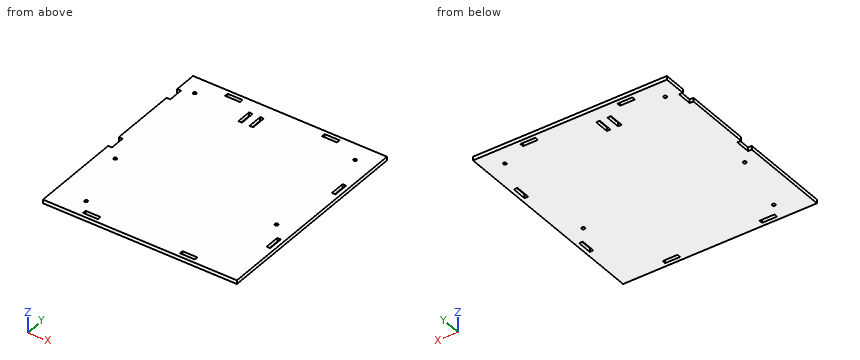
```python
from build123d import *

# Parameters (mm, degrees)
SKETCH1_W           = 260
SKETCH1_H           = 283
SKETCH1_W_2         = 20
SKETCH1_H_2         = 4.8
SKETCH1_W_3         = 4.8
SKETCH1_H_3         = 20
BOSS_EXTRUDE1_DEPTH = 5
SKETCH2_W           = 4.8
SKETCH2_H           = 20
CUT_EXTRUDE1_DEPTH  = 5
SKETCH3_R           = 2.1
CUT_EXTRUDE2_DEPTH  = 5
SKETCH4_R           = 2.1
CUT_EXTRUDE3_DEPTH  = 5
SKETCH5_R           = 2.1
CUT_EXTRUDE4_DEPTH  = 5
SKETCH6_R           = 2.1
CUT_EXTRUDE5_DEPTH  = 5
SKETCH7_W           = 5
SKETCH7_H           = 20
CUT_EXTRUDE6_DEPTH  = 10


with BuildPart() as part:
    # Sketch1 → Boss-Extrude1 (new body)
    with BuildSketch(Plane.XY):
        with Locations((-120, 136.5)):
            Rectangle(SKETCH1_W, SKETCH1_H)
        with Locations((-190, 2.5)):
            Rectangle(SKETCH1_W_2, SKETCH1_H_2, mode=Mode.SUBTRACT)
        with Locations((-60, 2.5)):
            Rectangle(SKETCH1_W_2, SKETCH1_H_2, mode=Mode.SUBTRACT)
        with Locations((2.5, 75)):
            Rectangle(SKETCH1_W_3, SKETCH1_H_3, mode=Mode.SUBTRACT)
        with Locations((2.5, 198)):
            Rectangle(SKETCH1_W_3, SKETCH1_H_3, mode=Mode.SUBTRACT)
        with Locations((-60, 270.5)):
            Rectangle(SKETCH1_W_2, SKETCH1_H_2, mode=Mode.SUBTRACT)
        with Locations((-190, 270.5)):
            Rectangle(SKETCH1_W_2, SKETCH1_H_2, mode=Mode.SUBTRACT)
    extrude(amount=BOSS_EXTRUDE1_DEPTH)

    # Sketch2 → Cut-Extrude1 (cut)
    with BuildSketch(Plane.XY.offset(5)):
        with Locations((-143.405234687, 248)):
            Rectangle(SKETCH2_W, SKETCH2_H)
        with Locations((-158.405234687, 248)):
            Rectangle(SKETCH2_W, SKETCH2_H)
    extrude(amount=-CUT_EXTRUDE1_DEPTH, mode=Mode.SUBTRACT)

    # Sketch3 → Cut-Extrude2 (cut)
    with BuildSketch(Plane.XY.offset(5)):
        with Locations((-230, 253)):
            Circle(SKETCH3_R)
        with Locations((-15, 253)):
            Circle(SKETCH3_R)
    extrude(amount=-CUT_EXTRUDE2_DEPTH, mode=Mode.SUBTRACT)

    # Sketch4 → Cut-Extrude3 (cut)
    with BuildSketch(Plane.XY.offset(5)):
        with Locations((-210, 20)):
            Circle(SKETCH4_R)
    extrude(amount=-CUT_EXTRUDE3_DEPTH, mode=Mode.SUBTRACT)

    # Sketch5 → Cut-Extrude4 (cut)
    with BuildSketch(Plane.XY.offset(5)):
        with Locations((-15, 105)):
            Circle(SKETCH5_R)
    extrude(amount=-CUT_EXTRUDE4_DEPTH, mode=Mode.SUBTRACT)

    # Sketch6 → Cut-Extrude5 (cut)
    with BuildSketch(Plane.XY.offset(5)):
        with Locations((-230, 103)):
            Circle(SKETCH6_R)
    extrude(amount=-CUT_EXTRUDE5_DEPTH, mode=Mode.SUBTRACT)

    # Sketch7 → Cut-Extrude6 (cut)
    with BuildSketch(Plane.XY.offset(5)):
        with Locations((-247.5, 238)):
            Rectangle(SKETCH7_W, SKETCH7_H)
        with Locations((-247.5, 128)):
            Rectangle(SKETCH7_W, SKETCH7_H)
    extrude(amount=-CUT_EXTRUDE6_DEPTH, mode=Mode.SUBTRACT)


solid = part.part
```
Model file for the job. Use its own axes, mm. Give positions to 0.01 mm unless a question says otherwise; leave off trailing zeros. Order: outer loops, then holes, each group sorted by start corner. A loop starts at its lowest first (then second) coordinate and runs counter-clockwise, first axis right, second up.
1) Wall check: probe 1 along Y at (x, z) = (-64, 3.7); probe 2 along Y at (x, z) = (-15, 3.9); probe 3 along X at (y, z) = (253, 3.05). Give the ranges that are in metal, low to high.
2) Saw through at A-A, the plane y = 81.5. Write the cut outline in (x, z), then the cut area to 3 significant figures.
3) Pin check, flat tip, straight feed: pin 1 (4 mm diameter, centred on x = -210, y = 20, fed in from -Z). Stop position of the tip, or through.
Computed:
1. probe 1: y = -5 to 0.1, 4.9 to 268.1, 272.9 to 278
1. probe 2: y = -5 to 102.9, 107.1 to 250.9, 255.1 to 278
1. probe 3: x = -250 to -232.1, -227.9 to -160.81, -156.01 to -145.81, -141.01 to -17.1, -12.9 to 10
2. outline: (-250, 0) - (0.1, 0) - (0.1, 5) - (-250, 5) - close; (4.9, 0) - (10, 0) - (10, 5) - (4.9, 5) - close
2. area: 1,280 mm2
3. pin 1: passes through
